Read the model definition and answer for the solid it produces. Units are mm, in the model's axes. Face numbers are marked on the shaded views. Round coordinates to 2 decimals unless told otherwise and drop trailing zeros. Loops run counter-clockwise (first coordinate to the right, second up) from the corner with the lowest first, then second, coordinate; pieces in that order, holes last. Notation, with made-up numbers: (-21, 74.25) -> (5, 74.25) arc R18 ccw to (5, 86.25) -> close; hole circle Ø5 at (52, -22.75). An arc over 180 degrees is marked (long way). Put each result on its own line as item: value.
from build123d import *

# Parameters (mm, degrees)
ESQUISSE1_R        = 15
ESQUISSE1_R_2      = 1.5
BOSS_EXTRU_1_DEPTH = 3


with BuildPart() as part:
    # Esquisse1 → Boss.-Extru.1 (new body)
    with BuildSketch(Plane(origin=(0, 0, 0), x_dir=(1, 0, 0), z_dir=(0, 1, 0))):
        Circle(ESQUISSE1_R)
        with Locations((-3.5, 0)):
            Circle(ESQUISSE1_R_2, mode=Mode.SUBTRACT)
        with Locations((3.5, 0)):
            Circle(ESQUISSE1_R_2, mode=Mode.SUBTRACT)
        with BuildLine():
            ThreePointArc((1.991071429, 2.878477821), (0.25, 0), (1.991071429, -2.878477821))
            ThreePointArc((1.991071429, -2.878477821), (0, -3.5), (-1.991071429, -2.878477821))
            ThreePointArc((-1.991071429, -2.878477821), (-0.25, 0), (-1.991071429, 2.878477821))
            ThreePointArc((-1.991071429, 2.878477821), (0, 3.5), (1.991071429, 2.878477821))
        make_face(mode=Mode.SUBTRACT)
    extrude(amount=BOSS_EXTRU_1_DEPTH)


solid = part.part
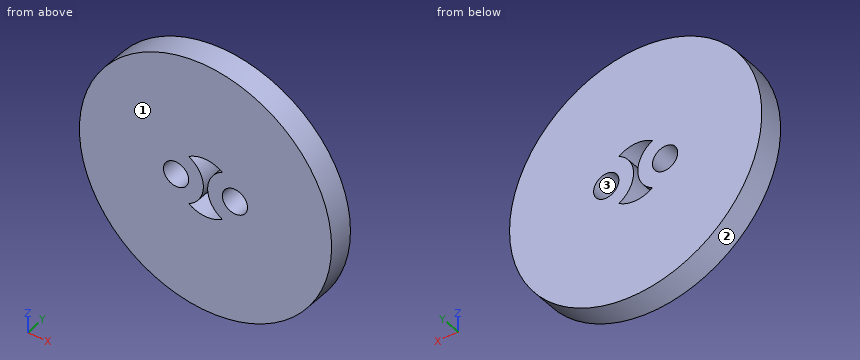
Item 1: Flat-ended cylindrical pins translate along their axes: pin 1 Ø1 at (x, z) = (12, 4.5) entering from -Y; pin 2 Ø1 at (y, z) = (2, 4.5) entering from +X. Find the tip coordinate at first contact, or state that the pin passes through.
Derived:
pin 1: stops at y = 0
pin 2: stops at x = 14.46
Item 2: For a pull along X with two mould halves and no side action, classify the marked faces 1, 2 and 3 as pulls with the +X half, pulls with the -X half, needs draft (parallel to the pull), parting line crosses it, or undercut.
Derived:
face 1: needs draft
face 2: parting line crosses it
face 3: undercut
Item 3: Find the intervals of material crossed by line 1 along X through (y, z) = (1.95, 0); line 2 along Z through (x, y) = (-0.75, 1.45); line 3 along Z through (x, y) = (3.5, 0.7), in increasing order.
Derived:
line 1: x = -15 to -5, -2 to -0.25, 0.25 to 2, 5 to 15
line 2: z = -14.98 to -3.42, -1.73 to 1.73, 3.42 to 14.98
line 3: z = -14.59 to -1.5, 1.5 to 14.59
Item 4: The part is cut by section C-C (y = 0.6). Determine the outline of the cut face in (x, z), then the cut area to 3 significant figures.
Derived:
outline: circle Ø30 at (0, 0); hole circle Ø3 at (-3.5, 0); hole (-1.99, -2.88) arc R3.5 ccw to (1.99, -2.88) arc R3.25 cw to (1.99, 2.88) arc R3.5 ccw to (-1.99, 2.88) arc R3.25 cw to start; hole circle Ø3 at (3.5, 0)
area: 681 mm^2
Item 5: The part is cut by section B-B (x = -2.5). Determine the outline of the cut face in (y, z), then the cut area to 3 significant figures.
Derived:
outline: (0, -14.79) -> (3, -14.79) -> (3, -1.12) -> (0, -1.12) -> close; (0, 1.12) -> (3, 1.12) -> (3, 14.79) -> (0, 14.79) -> close
area: 82.0 mm^2
Item 6: The part is cut by section A-A (z = 0). Determine the outline of the cut face in (x, y), then the cut area to 3 significant figures.
Derived:
outline: (-15, 0) -> (-5, 0) -> (-5, 3) -> (-15, 3) -> close; (-2, 0) -> (-0.25, 0) -> (-0.25, 3) -> (-2, 3) -> close; (0.25, 0) -> (2, 0) -> (2, 3) -> (0.25, 3) -> close; (5, 0) -> (15, 0) -> (15, 3) -> (5, 3) -> close
area: 70.5 mm^2
Item 7: The part is cut by section D-D (x = 4.5). Determine the outline of the cut face in (y, z), then the cut area to 3 significant figures.
Derived:
outline: (0, -14.31) -> (3, -14.31) -> (3, -1.12) -> (0, -1.12) -> close; (0, 1.12) -> (3, 1.12) -> (3, 14.31) -> (0, 14.31) -> close
area: 79.1 mm^2
